Verification items for the finished model (mm, model axes). Face numbers are marked on the shaded views. A direction names the side the tool comes from. Give positions to 0.01 mm unless a question says otherwise; leave off trailing zeros. Order: outer loops, then holes, each group sorted by start corner. A loop starts at its lowest first (then second) coordinate and runs counter-clockwise, first axis right, second up. Notation, with made-up numbers: M -17.5,38 L 19.5,38 A14 ccw 19.5,57 Z; hole C 2,-4 d3. An arc over 180 degrees is marked long. Answer as a JSON object with one key per item and string values.
```python
from build123d import *

# Parameters (mm, degrees)
PAD_DEPTH             = 4
PAD001_DEPTH          = 17
SKETCH002_W           = 2.5
SKETCH002_H           = 20
POCKET_DEPTH          = 3.4
POLARPATTERN_COUNT    = 4
SKETCH003_R           = 5
SKETCH003_W           = 44.642272
SKETCH003_H           = 44.642272
POCKET001_DEPTH       = 3.4
POLARPATTERN001_COUNT = 4
HOLE_D                = 5.2
HOLE_CBORE_D          = 10
HOLE_CBORE_DEPTH      = 13
SKETCH005_W           = 77.51
SKETCH005_H           = 1
POCKET002_DEPTH       = 19
POLARPATTERN002_COUNT = 4
CHAMFER_SIZE          = 1
SKETCH006_R           = 1.55
HOLE001_DEPTH         = 14.068666
HOLE001_TIPS_R        = 1.55
CHAMFER001_SIZE       = 1
CHAMFER001_FACE140_W  = 0.9
CHAMFER001_FACE140_H  = 15
PAD002_DEPTH          = 5
PAD002_FACE143_W      = 15
PAD002_FACE143_H      = 0.9
PAD003_DEPTH          = 5
PAD003_FACE75_W       = 15
PAD003_FACE75_H       = 0.9
PAD004_DEPTH          = 5
PAD004_FACE128_W      = 0.9
PAD004_FACE128_H      = 15
PAD005_DEPTH          = 5


with BuildPart() as part:
    # Sketch → Pad (new body)
    with BuildSketch(Plane.XY):
        with BuildLine():
            Line((-50, 55), (50, 55))
            ThreePointArc((55, 50), (53.535534, 53.535534), (50, 55))
            Line((55, 50), (55, -50))
            ThreePointArc((50, -55), (53.535534, -53.535534), (55, -50))
            Line((50, -55), (-50, -55))
            ThreePointArc((-55, -50), (-53.535534, -53.535534), (-50, -55))
            Line((-55, -50), (-55, 50))
            ThreePointArc((-50, 55), (-53.535534, 53.535534), (-55, 50))
        make_face()
    extrude(amount=PAD_DEPTH)

    # Sketch001 (on Face9 of Pad) → Pad001 (join)
    with BuildSketch(Plane(origin=(0, 0, 0), x_dir=(1, 0, 0), z_dir=(0, 0, -1))):
        Polygon((-51.4, 40), (-48.7, 40), (-48.7, 47.7), (-47.7, 48.7), (-40, 48.7), (-40, 51.4), (-7.5, 51.4), (-7.5, 49.5), (7.5, 49.5), (7.5, 51.4), (40, 51.4), (40, 48.7), (47.7, 48.7), (48.7, 47.7), (48.7, 40), (51.4, 40), (51.4, 7.5), (49.5, 7.5), (49.5, -7.5), (51.4, -7.5), (51.4, -40), (48.7, -40), (48.7, -47.7), (47.7, -48.7), (40, -48.7), (40, -51.4), (7.5, -51.4), (7.5, -49.5), (-7.5, -49.5), (-7.5, -51.4), (-40, -51.4), (-40, -48.7), (-47.7, -48.7), (-48.7, -47.7), (-48.7, -40), (-51.4, -40), (-51.4, -7.5), (-49.5, -7.5), (-49.5, 7.5), (-51.4, 7.5), align=None)
    extrude(amount=PAD001_DEPTH)

    # Sketch002 (on Face51 of Pad001) → Pocket (cut)
    with BuildSketch(Plane(origin=(0, 0, -17), x_dir=(1, 0, 0), z_dir=(0, 0, -1))):
        with Locations((-40.005, 56)):
            Rectangle(SKETCH002_W, SKETCH002_H)
        with Locations((-13.335, 56)):
            Rectangle(SKETCH002_W, SKETCH002_H)
        with Locations((13.335, 56)):
            Rectangle(SKETCH002_W, SKETCH002_H)
        with Locations((40.005, 56)):
            Rectangle(SKETCH002_W, SKETCH002_H)
    pocket = extrude(amount=-POCKET_DEPTH, mode=Mode.SUBTRACT)

    # PolarPattern: Pocket ×4 about axis
    polarpattern_axis = Axis((0, 0, 0), (0, 0, 1))
    for i in range(1, POLARPATTERN_COUNT):
        add(pocket.rotate(polarpattern_axis, i * 360 / POLARPATTERN_COUNT), mode=Mode.SUBTRACT)

    # Sketch003 (on Face52 of PolarPattern) → Pocket001 (cut)
    with BuildSketch(Plane(origin=(0, 0, -17), x_dir=(1, 0, 0), z_dir=(0, 0, -1))):
        with Locations((-26.67, 26.67)):
            Circle(SKETCH003_R)
        with Locations((-61.076136, 61.076136)):
            Rectangle(SKETCH003_W, SKETCH003_H)
    pocket001 = extrude(amount=-POCKET001_DEPTH, mode=Mode.SUBTRACT)

    # PolarPattern001: Pocket001 ×4 about axis
    polarpattern001_axis = Axis((0, 0, 0), (0, 0, 1))
    for i in range(1, POLARPATTERN001_COUNT):
        add(pocket001.rotate(polarpattern001_axis, i * 360 / POLARPATTERN001_COUNT), mode=Mode.SUBTRACT)

    # Hole (through all)
    with Locations(Plane(origin=(0, 0, -17), x_dir=(1, 0, 0), z_dir=(0, 0, -1))):
        with Locations((-22.225, 42.5), (22.225, 42.5), (22.225, -42.5), (-22.225, -42.5)):
            CounterBoreHole(HOLE_D / 2, HOLE_CBORE_D / 2, HOLE_CBORE_DEPTH)

    # Sketch005 (on Face56 of Hole) → Pocket002 (cut)
    with BuildSketch(Plane(origin=(0, 0, -17), x_dir=(1, 0, 0), z_dir=(0, 0, -1))):
        with Locations((0, 50.9)):
            Rectangle(SKETCH005_W, SKETCH005_H)
    pocket002 = extrude(amount=-POCKET002_DEPTH, mode=Mode.SUBTRACT)

    # PolarPattern002: Pocket002 ×4 about axis
    polarpattern002_axis = Axis((0, 0, 0), (0, 0, 1))
    for i in range(1, POLARPATTERN002_COUNT):
        add(pocket002.rotate(polarpattern002_axis, i * 360 / POLARPATTERN002_COUNT), mode=Mode.SUBTRACT)

    # Chamfer
    chamfer_edges = [part.edges().sort_by_distance(p)[0] for p in [
        (51.4, 0, 0),
        (0, -51.4, 0),
        (-51.4, 0, 0),
        (0, 51.4, 0),
    ]]
    chamfer(chamfer_edges, length=CHAMFER_SIZE)

    # Sketch006 (on Face75 of Chamfer) → Hole001 (cut)
    with BuildSketch(Plane(origin=(0, 0, -17), x_dir=(1, 0, 0), z_dir=(0, 0, -1))):
        with Locations((-44, 44)):
            Circle(SKETCH006_R)
        with Locations((44, 44)):
            Circle(SKETCH006_R)
        with Locations((44, -44)):
            Circle(SKETCH006_R)
        with Locations((-44, -44)):
            Circle(SKETCH006_R)
        Circle(SKETCH006_R)
    extrude(amount=-HOLE001_DEPTH, mode=Mode.SUBTRACT)

    # Hole001 tips → Hole001 tip 1 section 0
    with BuildSketch(Plane(origin=(0, 0, -2.931334), x_dir=(1, 0, 0), z_dir=(0, 0, -1)), mode=Mode.PRIVATE) as hole001_tip_1_s0:
        with Locations((-44, 44)):
            Circle(HOLE001_TIPS_R)
    loft([hole001_tip_1_s0.sketch, Vertex(-44, -44, -2)], mode=Mode.SUBTRACT)

    # Hole001 tips → Hole001 tip 2 section 0
    with BuildSketch(Plane(origin=(0, 0, -2.931334), x_dir=(1, 0, 0), z_dir=(0, 0, -1)), mode=Mode.PRIVATE) as hole001_tip_2_s0:
        with Locations((44, 44)):
            Circle(HOLE001_TIPS_R)
    loft([hole001_tip_2_s0.sketch, Vertex(44, -44, -2)], mode=Mode.SUBTRACT)

    # Hole001 tips → Hole001 tip 3 section 0
    with BuildSketch(Plane(origin=(0, 0, -2.931334), x_dir=(1, 0, 0), z_dir=(0, 0, -1)), mode=Mode.PRIVATE) as hole001_tip_3_s0:
        with Locations((44, -44)):
            Circle(HOLE001_TIPS_R)
    loft([hole001_tip_3_s0.sketch, Vertex(44, 44, -2)], mode=Mode.SUBTRACT)

    # Hole001 tips → Hole001 tip 4 section 0
    with BuildSketch(Plane(origin=(0, 0, -2.931334), x_dir=(1, 0, 0), z_dir=(0, 0, -1)), mode=Mode.PRIVATE) as hole001_tip_4_s0:
        with Locations((-44, -44)):
            Circle(HOLE001_TIPS_R)
    loft([hole001_tip_4_s0.sketch, Vertex(-44, 44, -2)], mode=Mode.SUBTRACT)

    # Hole001 tips → Hole001 tip 5 section 0
    with BuildSketch(Plane(origin=(0, 0, -2.931334), x_dir=(1, 0, 0), z_dir=(0, 0, -1)), mode=Mode.PRIVATE) as hole001_tip_5_s0:
        Circle(HOLE001_TIPS_R)
    loft([hole001_tip_5_s0.sketch, Vertex(0, 0, -2)], mode=Mode.SUBTRACT)

    # Chamfer001
    chamfer001_edges = [part.edges().sort_by_distance(p)[0] for p in [
        (1.55, 0, -17),
        (-42.45, 44, -13.6),
        (-42.45, -44, -13.6),
        (45.55, 44, -13.6),
        (45.55, -44, -13.6),
    ]]
    chamfer(chamfer001_edges, length=CHAMFER001_SIZE)

    # Chamfer001 Face140 → Pad002 (add)
    with BuildSketch(Plane(origin=(0, 49.95, 0), x_dir=(0, -1, 0), z_dir=(0, 0, -1))):
        Rectangle(CHAMFER001_FACE140_W, CHAMFER001_FACE140_H)
    extrude(amount=PAD002_DEPTH)

    # Pad002 Face143 → Pad003 (add)
    with BuildSketch(Plane(origin=(-49.95, 0, 0), x_dir=(0, -1, 0), z_dir=(0, 0, -1))):
        Rectangle(PAD002_FACE143_W, PAD002_FACE143_H)
    extrude(amount=PAD003_DEPTH)

    # Pad003 Face75 → Pad004 (add)
    with BuildSketch(Plane(origin=(49.95, 0, 0), x_dir=(0, -1, 0), z_dir=(0, 0, -1))):
        Rectangle(PAD003_FACE75_W, PAD003_FACE75_H)
    extrude(amount=PAD004_DEPTH)

    # Pad004 Face128 → Pad005 (add)
    with BuildSketch(Plane(origin=(0, -49.95, 0), x_dir=(0, -1, 0), z_dir=(0, 0, -1))):
        Rectangle(PAD004_FACE128_W, PAD004_FACE128_H)
    extrude(amount=PAD005_DEPTH)


solid = part.part
```
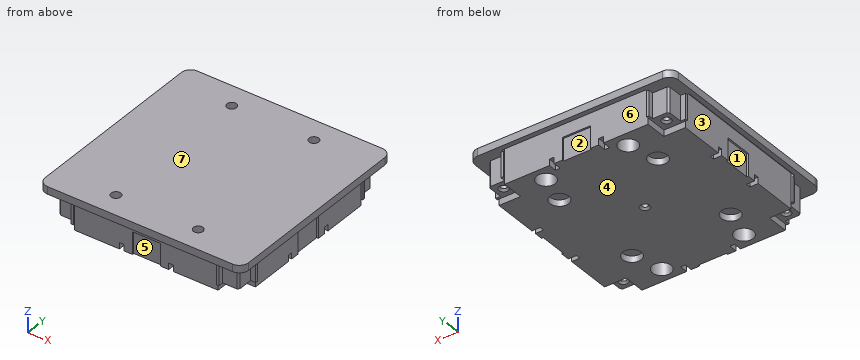
Q1. Material ranges on L1, parallel to X at y = -42.5, z = 2.25 (3 decimals); L2, parallel to Y at x = -20, z = -8.25; L3, parallel to X at y = -42.5, z = -1.75 (3 decimals), recorded low to high.
Resolved:
{"L1": "x = -55 to -24.825, -19.625 to 19.625, 24.825 to 55", "L2": "y = -50.4 to -46.98, -38.02 to 38.02, 46.98 to 50.4", "L3": "x = -48.7 to -24.825, -19.625 to 19.625, 24.825 to 48.7"}
Q2. Section check D-D on y = -28. Record the cut outline in (x, z).
Resolved:
{"outline": "M -55,0 L -52.4,0 L -51.4,1 L -51.4,2 L -50.4,2 L -50.4,-17 L -31.49,-17 L -31.49,-13.6 L -21.85,-13.6 L -21.85,-17 L 21.85,-17 L 21.85,-13.6 L 31.49,-13.6 L 31.49,-17 L 50.4,-17 L 50.4,2 L 51.4,2 L 51.4,1 L 52.4,0 L 55,0 L 55,4 L -55,4 Z"}
Q3. Section check A-A on x = -4. Record the cut outline in (y, z), then the cut area to 3 significant figures.
Resolved:
{"outline": "M -55,0 L -52.4,0 L -51.4,1 L -51.4,2 L -50.4,2 L -50.4,-5 L -49.5,-5 L -49.5,-17 L 49.5,-17 L 49.5,-5 L 50.4,-5 L 50.4,2 L 51.4,2 L 51.4,1 L 52.4,0 L 55,0 L 55,4 L -55,4 Z", "area": "2,130 mm²"}
Q4. Release check for a two-part mould opening along X. For the marked faces 1, 2, 3 and 4 record: +X half, -X half, draft (parallel to the pull), parting line (faces both ways), or undercut.
Resolved:
{"face 1": "-X half", "face 2": "undercut", "face 3": "undercut", "face 4": "draft"}
Q5. Gauge pin test, flat ends, axial feed: pin 1 Ø6 at (x, z) = (-19.5, -10.5) entering from +Y; pin 2 Ø10 at (x, z) = (-13, -13.5) entering from -Y; pin 3 Ø1.2 at (x, z) = (13.5, -15.5) entering from -Y. Record the tip position at first contact, or that the pin passes through.
Resolved:
{"pin 1": "stops at y = 50.4", "pin 2": "stops at y = -50.4", "pin 3": "stops at y = -46"}
Q6. Section check B-B on y = 26.67. Record the cut outline in (x, z), then the cut area to 3 significant figures.
Resolved:
{"outline": "M -55,0 L -52.4,0 L -51.4,1 L -51.4,2 L -50.4,2 L -50.4,-17 L -31.67,-17 L -31.67,-13.6 L -21.67,-13.6 L -21.67,-17 L 21.67,-17 L 21.67,-13.6 L 31.67,-13.6 L 31.67,-17 L 50.4,-17 L 50.4,2 L 51.4,2 L 51.4,1 L 52.4,0 L 55,0 L 55,4 L -55,4 Z", "area": "2,080 mm²"}
Q7. Tool access check on the marked faces 5, 6 and 7. Record the directions out of +Z, -Z, +X, -X, +Y, -Y that give a thin tool (end or side, any length) a straight path to the whole face; none if there is none.
Resolved:
{"face 5": "-Z, -Y", "face 6": "-Z", "face 7": "+Z, +X, -X, +Y, -Y"}
Q8. Section check C-C on z = -7.5. Count the separate pieces of the cut face and the enclosed holes in it, then the cut area to 3 significant figures.
Resolved:
{"separate pieces": "1", "enclosed holes": "9", "area": "9,630 mm²"}
